Work out the finished part from the listing and answer in its coordinate system (mm). A direction names the side the tool comes from. Coordinates: 2 decimals unless noted, no trailing zeros. Order: outer loops, then holes, each group sorted by start corner. A loop starts at its lowest first (then second) coordinate and runs counter-clockwise, first axis right, second up. Notation, with made-up numbers: M 39,-12 L 78,-12 A34 ccw 78,22 Z; hole C -27,54 d6. An arc over 180 degrees is marked long. Answer in a Markdown table with one row per item. Add a question column.
Item 1: Consider line 1 (Y direction, x = 7.75, z = 6); line 2 (Y direction, x = 8.5, z = 2); line 3 (X direction, y = 29, z = 10.5). Determine where each line is inside the solid, lowest interval first. Write a range as from..to.
Item 2: A flat-ended cylindrical pin translates along its axis: pin 1 Ø3 at (x, y) = (11, 29) entering from +Z. Find the tip coordinate at first contact, or state that the pin passes through.
Item 3: The part is cut by section A-A (z = 9). Write down the section's boundary in (x, y).
Item 4: The part is cut by section B-B (y = 23.75). Write down the section's boundary in (x, z).
Item 5: The part is cut by section C-C (x = 8.5). Write down the section's boundary in (y, z), then the cut area to 3 significant figures.
Item 6: The part is cut by section D-D (y = 21.5). Write down the section's boundary in (x, z), then the cut area to 3 significant figures.
Item 7: The mould has two halves that part along Y. Classify faces 1 (the face through (7.28, 24.93, 5.19)), 2 (the face through (1.78, 28, 6)), 3 (the face through (6, 35.847, 5)), 4 (the face through (6, 20.347, 5)): released by +Y, released by -Y, zero draft, split by the parting line, or undercut.
Item 8: Which of the six approach directions +Z, -Z, +X, -X, +Y, -Y give full straight-line access (tool end or side, diameter ignored) to faces 5 (the face through (3.808, 33.334, 8.195)), 6 (the face through (12, 28, 4)), 7 (the face through (7, 24.8, 5.5))?
from build123d import *

# Parameters (mm, degrees)
SKETCH1_W           = 12
SKETCH1_H           = 15.5
BOSS_EXTRUDE1_DEPTH = 4
SKETCH2_W           = 4
SKETCH2_H           = 15.5
BOSS_EXTRUDE2_DEPTH = 8.5
SKETCH3_R           = 1.5
CUT_EXTRUDE1_DEPTH  = 5
SKETCH4_R           = 1.5
CUT_EXTRUDE2_DEPTH  = 5
BOSS_EXTRUDE3_DEPTH = 15.5
SKETCH6_R           = 2.5
CUT_EXTRUDE3_DEPTH  = 8
SKETCH7_R           = 2.5
CUT_EXTRUDE4_DEPTH  = 8.5


with BuildPart() as part:
    # Sketch1 → Boss-Extrude1 (new body)
    with BuildSketch(Plane.XY):
        with Locations((7.780385216, 28.096978354)):
            Rectangle(SKETCH1_W, SKETCH1_H)
    extrude(amount=BOSS_EXTRUDE1_DEPTH)

    # Sketch2 → Boss-Extrude2 (add)
    with BuildSketch(Plane.XY.offset(4)):
        with Locations((3.780385216, 28.096978354)):
            Rectangle(SKETCH2_W, SKETCH2_H)
    extrude(amount=BOSS_EXTRUDE2_DEPTH)

    # Sketch3 → Cut-Extrude1 (cut)
    with BuildSketch(Plane(origin=(5.780385216, 0, 0), x_dir=(0, 0, -1), z_dir=(1, 0, 0))):
        with Locations((-8, 24.846978354)):
            Circle(SKETCH3_R)
        with Locations((-8, 31.846978354)):
            Circle(SKETCH3_R)
    extrude(amount=-CUT_EXTRUDE1_DEPTH, mode=Mode.SUBTRACT)

    # Sketch4 → Cut-Extrude2 (cut)
    with BuildSketch(Plane.XY.offset(4)):
        with Locations((9.780385216, 24.846978354)):
            Circle(SKETCH4_R)
        with Locations((9.780385216, 31.846978354)):
            Circle(SKETCH4_R)
    extrude(amount=-CUT_EXTRUDE2_DEPTH, mode=Mode.SUBTRACT)

    # Sketch5 → Boss-Extrude3 (add)
    with BuildSketch(Plane(origin=(0, 35.846978354, 0), x_dir=(1, 0, 0), z_dir=(0, 1, 0))):
        Polygon((5.780385216, -4), (5.780385216, -10), (11.780385216, -4), align=None)
    extrude(amount=-BOSS_EXTRUDE3_DEPTH)

    # Sketch6 → Cut-Extrude3 (cut)
    with BuildSketch(Plane(origin=(13.780385216, 0, 0), x_dir=(0, 0, -1), z_dir=(1, 0, 0))):
        with Locations((-8, 31.846978354)):
            Circle(SKETCH6_R)
        with Locations((-8, 24.846978354)):
            Circle(SKETCH6_R)
    extrude(amount=-CUT_EXTRUDE3_DEPTH, mode=Mode.SUBTRACT)

    # Sketch7 → Cut-Extrude4 (cut)
    with BuildSketch(Plane.XY.offset(12.5)):
        with Locations((9.780385216, 31.846978354)):
            Circle(SKETCH7_R)
        with Locations((9.780385216, 24.846978354)):
            Circle(SKETCH7_R)
    extrude(amount=-CUT_EXTRUDE4_DEPTH, mode=Mode.SUBTRACT)


solid = part.part
Reply:
| question | item | result |
|---|---|---|
| 1 | line 1 | y = 20.35..23.35, 26.35..30.35, 33.35..35.85 |
| 1 | line 2 | y = 20.35..24.07, 25.63..31.07, 32.63..35.85 |
| 1 | line 3 | x = 1.78..5.78 |
| 2 | pin 1 | stops at z = 6.28 |
| 3 | outline | M 1.78,20.35 L 6.78,20.35 L 6.78,22.56 L 5.78,22.56 L 5.78,23.73 L 1.78,23.73 Z; M 1.78,25.97 L 5.78,25.97 L 5.78,27.14 L 6.78,27.14 L 6.78,29.56 L 5.78,29.56 L 5.78,30.73 L 1.78,30.73 Z; M 1.78,32.97 L 5.78,32.97 L 5.78,34.14 L 6.78,34.14 L 6.78,35.85 L 1.78,35.85 Z |
| 4 | outline | M 1.78,0 L 8.76,0 L 8.76,4 L 7.53,4 L 7.53,5.75 L 5.78,5.75 L 5.78,6.98 L 1.78,6.98 Z; M 1.78,9.02 L 5.78,9.02 L 5.78,12.5 L 1.78,12.5 Z; M 10.8,0 L 13.78,0 L 13.78,4 L 10.8,4 Z |
| 5 | outline | M 20.35,0 L 24.07,0 L 24.07,4 L 22.7,4 L 22.7,6.72 A2.5 cw 22.45,7.28 L 20.35,7.28 Z; M 25.63,0 L 31.07,0 L 31.07,4 L 29.7,4 L 29.7,6.72 A2.5 cw 29.45,7.28 L 27.24,7.28 A2.5 cw 26.99,6.72 L 26.99,4 L 25.63,4 Z; M 32.63,0 L 35.85,0 L 35.85,7.28 L 34.24,7.28 A2.5 cw 33.99,6.72 L 33.99,4 L 32.63,4 Z |
| 5 | area | 71.9 mm2 |
| 6 | outline | M 1.78,0 L 13.78,0 L 13.78,4 L 11.78,4 L 5.78,10 L 5.78,12.5 L 1.78,12.5 Z |
| 6 | area | 100 mm2 |
| 7 | face 1 | undercut |
| 7 | face 2 | zero draft |
| 7 | face 3 | released by +Y |
| 7 | face 4 | released by -Y |
| 8 | face 5 | +X, -X |
| 8 | face 6 | +Z |
| 8 | face 7 | +X |
